Input: part model. Units: mm. Frame: model coordinates. Face numbers are marked on the shaded views. A direction names the side the tool comes from. Round coordinates to 2 decimals unless told otherwise and drop trailing zeros. Loops run counter-clockwise (first coordinate to the right, second up) from the corner with the lowest first, then second, coordinate; pieces in that order, holes last. Notation, with made-up numbers: (7.25, -31) -> (61.25, -31) arc R20 cw to (61.25, -26) -> close; hole circle Ø5 at (43, 32.5). An arc over 180 degrees is marked (long way). Answer as a JSON object with one key per item and string values. Group by question number.
Item 1: Section query D-D on z = -3.5. Return loops of the section in (x, y).
Item 2: Set-up query: the marked faces 4, 5 and 6. Return all of +Z, -Z, +X, -X, +Y, -Y with unobstructed straight access to the full face (end or side cutting, diameter ignored); none if empty.
Item 3: Pin query (flat end, axial travel): pin 1 (2 mm diameter, centred on x = 0, z = 33.95, fed in from +Y); pin 2 (9.5 mm diameter, centred on x = 0, z = -33.95, fed in from -Y); pin 3 (1.5 mm diameter, centred on y = 12.5, z = -6.5, fed in from -X); pin 4 (2 mm diameter, centred on y = 15.5, z = 12, fed in from -X). Return the tip coordinate at first contact, or that it passes through.
Item 4: Material intervals for line 1 (Z direction, x = -0.5, y = 12.5); line 2 (Y direction, x = 23.5, z = 5); line 3 (X direction, y = 5.5, z = -26), sorted ascending. Write a range as [from, to].
Item 5: Section query C-C on z = 33.95. Return loops of the section in (x, y).
Item 6: Section query B-B on y = 6.25. Return loops of the section in (x, z).
Item 7: Draft query along Z for the marked faces 1, 2 and 3. Return one class per face: released by +Z, released by -Z, zero draft, split by the parting line, or undercut.
Item 8: Section query A-A on x = -14.5. Return loops of the section in (y, z).
from build123d import *

# Parameters (mm, degrees)
BOSS_EXTRUDE3_DEPTH = 16.5
BOSS_EXTRUDE5_DEPTH = 1.5
SKETCH13_R          = 31
CUT_EXTRUDE1_DEPTH  = 8
SKETCH14_R          = 29
CUT_EXTRUDE2_DEPTH  = 8
M3_TAPPED_HOLE1_D   = 2.5
CIRPATTERN1_COUNT   = 3
HOLE1_D             = 3.5
HOLE1_DEPTH         = 18
HOLE1_CBORE_D       = 6
HOLE1_CBORE_DEPTH   = 4
CIRPATTERN2_COUNT   = 2


with BuildPart() as part:
    # Sketch7 → Boss-Extrude3 (new body)
    with BuildSketch(Plane(origin=(0, 0, 0), x_dir=(1, 0, 0), z_dir=(0, 1, 0))):
        with BuildLine():
            Line((17.663521733, 37), (-17.663521733, 37))
            ThreePointArc((-17.663521733, 37), (-28.858964332, 29.123189689), (-36.837480913, 18))
            Line((-36.837480913, 18), (3.3e-08, 18))
            Line((3.3e-08, 18), (36.837480913, 18))
            ThreePointArc((36.837480913, 18), (28.858964332, 29.123189689), (17.663521733, 37))
        make_face()
        with BuildLine():
            Line((0, -18), (36.837480913, -18))
            Line((36.837480913, -18), (36.837480913, 18))
            Line((36.837480913, 18), (3.3e-08, 18))
            ThreePointArc((3.3e-08, 18), (12.727922073, 12.72792205), (18, 0))
            ThreePointArc((18, 0), (12.727922061, -12.727922061), (0, -18))
        make_face()
        with BuildLine():
            Line((36.837480913, 18), (36.837480913, -18))
            ThreePointArc((36.837480913, -18), (39.945817787, -9.237512722), (41, 0))
            ThreePointArc((41, 0), (39.945817787, 9.237512722), (36.837480913, 18))
        make_face()
        with BuildLine():
            ThreePointArc((-36.837480913, -18), (-28.858964332, -29.123189689), (-17.663521733, -37))
            Line((-17.663521733, -37), (17.663521733, -37))
            ThreePointArc((17.663521733, -37), (28.858964332, -29.123189689), (36.837480913, -18))
            Line((36.837480913, -18), (0, -18))
            Line((0, -18), (-36.837480913, -18))
        make_face()
    extrude(amount=BOSS_EXTRUDE3_DEPTH)

    # Sketch11 → Boss-Extrude5 (add)
    with BuildSketch(Plane(origin=(0, 16.5, 0), x_dir=(1, 0, 0), z_dir=(0, 1, 0))):
        with BuildLine():
            Line((-32.32645975, 18), (0, 18))
            ThreePointArc((0, 18), (12.727922061, 12.727922061), (18, 0))
            ThreePointArc((18, 0), (12.727922061, -12.727922061), (0, -18))
            Line((0, -18), (-32.32645975, -18))
            ThreePointArc((-32.32645975, -18), (9.298413554, -35.812560721), (37, 0))
            ThreePointArc((37, 0), (9.298413554, 35.812560721), (-32.32645975, 18))
        make_face()
    extrude(amount=BOSS_EXTRUDE5_DEPTH)

    # Sketch13 → Cut-Extrude1 (cut)
    with BuildSketch(Plane(origin=(0, 18, 0), x_dir=(1, 0, 0), z_dir=(0, 1, 0))):
        Circle(SKETCH13_R)
    extrude(amount=-CUT_EXTRUDE1_DEPTH, mode=Mode.SUBTRACT)

    # Sketch14 → Cut-Extrude2 (cut)
    with BuildSketch(Plane.XZ):
        Circle(SKETCH14_R)
    extrude(amount=-CUT_EXTRUDE2_DEPTH, mode=Mode.SUBTRACT)

    # M3 Tapped Hole1 (through all)
    with Locations(Plane(origin=(35, 0, 0), x_dir=(0, 0, -1), z_dir=(0, -1, 0))):
        with Locations((0, 0)):
            m3_tapped_hole1 = Hole(M3_TAPPED_HOLE1_D / 2)

    # CirPattern1: M3 Tapped Hole1 ×3 about axis
    cirpattern1_axis = Axis((0, 0, 0), (0, 1, 0))
    for i in range(1, CIRPATTERN1_COUNT):
        add(m3_tapped_hole1.rotate(cirpattern1_axis, i * 360 / CIRPATTERN1_COUNT), mode=Mode.SUBTRACT)

    # Hole1
    with Locations(Plane(origin=(0, 0, 33.95), x_dir=(0, 0, -1), z_dir=(0, -1, 0))):
        with Locations((0, 0), (30.604436826, -13.912164411)):
            hole1 = CounterBoreHole(HOLE1_D / 2, HOLE1_CBORE_D / 2, HOLE1_CBORE_DEPTH, depth=HOLE1_DEPTH)

    # CirPattern2: Hole1 ×2 about axis
    cirpattern2_axis = Axis((0, 0, 0), (0, 1, 0))
    for i in range(1, CIRPATTERN2_COUNT):
        add(hole1.rotate(cirpattern2_axis, i * 360 / CIRPATTERN2_COUNT), mode=Mode.SUBTRACT)


solid = part.part
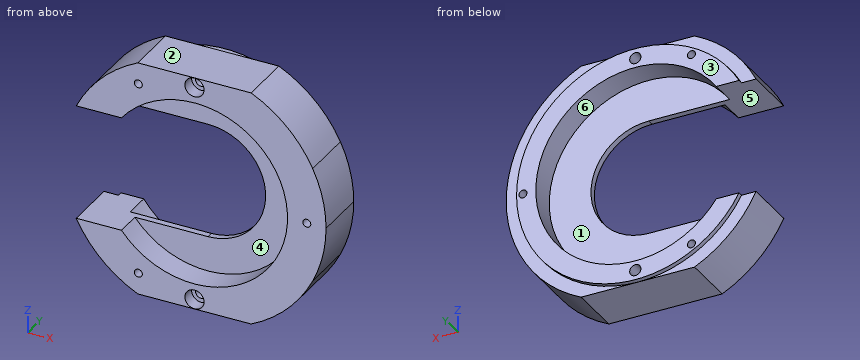
Solved:
{
 "1": {"outline": "(17.66, 8) -> (28.79, 8) -> (28.79, 0) -> (40.85, 0) -> (40.85, 16.5) -> (36.83, 16.5) -> (36.83, 18) -> (30.8, 18) -> (30.8, 10) -> (17.66, 10) -> close"},
 "2": {"face 4": "-Y", "face 5": "-X, +Y, -Y", "face 6": "+Y"},
 "3": {"pin 1": "through", "pin 2": "y = 0", "pin 3": "x = 30.14", "pin 4": "x = 28.14"},
 "4": {"line 1": "[-37, -35.63], [-32.27, -31], [31, 32.27], [35.63, 37]", "line 2": "[8, 10]", "line 3": "[-31.7, -12.85], [12.85, 31.7]"},
 "5": {"outline": "(-22.99, 0) -> (-3, 0) -> (-3, 4) -> (-1.75, 4) -> (-1.75, 18) -> (-14.71, 18) -> (-14.71, 16.5) -> (-22.99, 16.5) -> close; (1.75, 4) -> (3, 4) -> (3, 0) -> (22.99, 0) -> (22.99, 16.5) -> (14.71, 16.5) -> (14.71, 18) -> (1.75, 18) -> close"},
 "6": {"outline": "(-36.84, -18) arc R41 ccw to (-17.66, -37) -> (17.66, -37) arc R41 ccw to (17.66, 37) -> (-17.66, 37) arc R41 ccw to (-36.84, 18) -> (-22.74, 18) arc R29 cw (long way) to (-22.74, -18) -> close; hole circle Ø2.5 at (-17.5, -30.31); hole circle Ø2.5 at (-17.5, 30.31); hole circle Ø3.5 at (0, -33.95); hole circle Ø3.5 at (0, 33.95); hole circle Ø2.5 at (35, 0)"},
 "7": {"face 1": "undercut", "face 2": "released by +Z", "face 3": "zero draft"},
 "8": {"outline": "(0, -37) -> (16.5, -37) -> (16.5, -34.04) -> (18, -34.04) -> (18, -27.4) -> (10, -27.4) -> (10, -18) -> (8, -18) -> (8, -25.11) -> (0, -25.11) -> close; (0, 25.11) -> (8, 25.11) -> (8, 18) -> (10, 18) -> (10, 27.4) -> (18, 27.4) -> (18, 34.04) -> (16.5, 34.04) -> (16.5, 37) -> (0, 37) -> close"}
}
